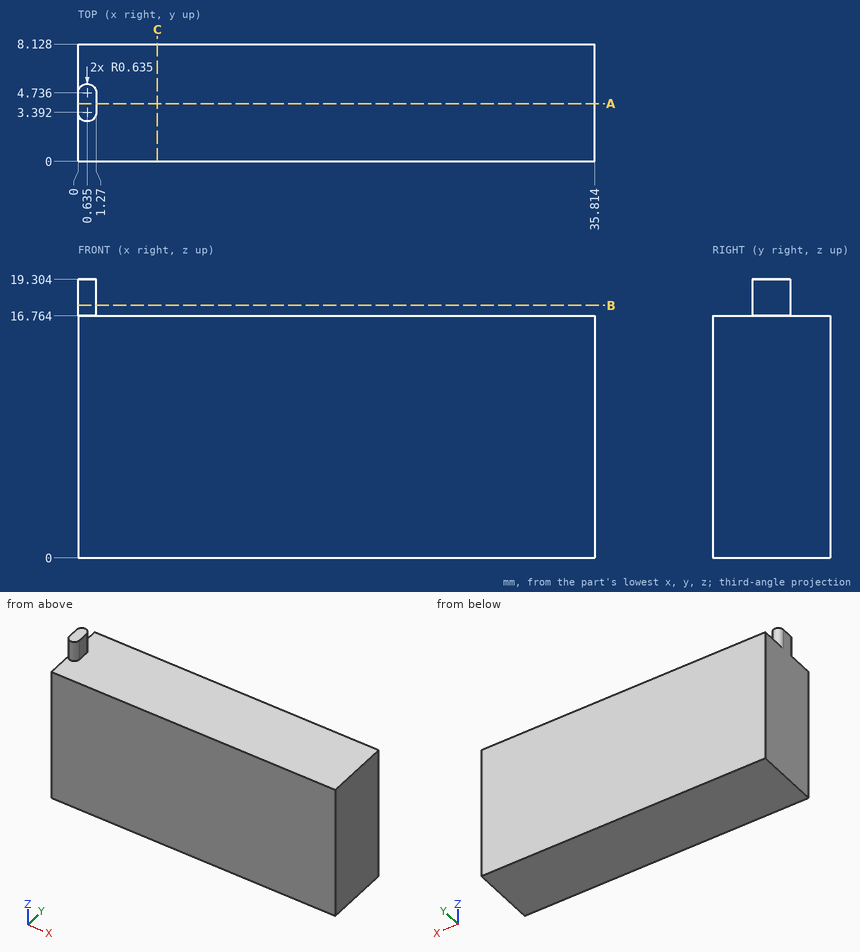
Geometry check sheet. Reference: drawing and pictorial views, mm from the part's lowest x, y, z. Give positions to 0.01 mm unless a question says otherwise; leave off trailing zeros. Write each loop counter-clockwise with the first axis right and the second up, starting at its lowest first coordinate (ties: lowest second). Pieces come first, ordered by that corner, then holes.
Item 1: Cross-section at A-A (y = 4). Enter the section's corners in (x, z).
Item 2: Cross-section at B-B (z = 17.5). Enter the section's corners in (x, y) (1 decimal).
Item 3: Gauge pin test, flat end, axial feed: pin 1 (2.5 mm diameter, centred on x = 14.5, y = 4, fed in from +Z). Record the tip position at first contact, or that the pin passes through.
Item 4: Cross-section at C-C (x = 5.5). Enter the section's corners in (y, z), and give its area (3 significant figures).
Item 5: Scan line: L1, parallel to Z at x = 9, y = 3.25. Record every from-to range of solid material in increasing order.
Report:
1. outline: (0, 0) - (35.81, 0) - (35.81, 16.76) - (1.27, 16.76) - (1.27, 19.3) - (0, 19.3) - close
2. outline: (0, 3.4) arc R0.6 ccw to (1.3, 3.4) - (1.3, 4.7) arc R0.6 ccw to (0, 4.7) - close
3. pin 1: stops at z = 16.76
4. outline: (0, 0) - (8.13, 0) - (8.13, 16.76) - (0, 16.76) - close
4. area: 136 mm2
5. L1: z = 0 to 16.76
